Part model, mm, in its own coordinate system. Face numbers are marked on the shaded views. A direction names the side the tool comes from. Give positions to 0.01 mm unless a question says otherwise; leave off trailing zeros. Loops run counter-clockwise (first coordinate to the right, second up) from the corner with the lowest first, then second, coordinate; pieces in that order, holes last. Notation, with made-up numbers: (34.25, -8.75) -> (82.25, -8.75) arc R17 cw to (82.25, 14.25) -> close; hole circle Ø4 at (48, -8). An arc over 180 degrees is marked (long way). One line per question, with ' | ' between items.
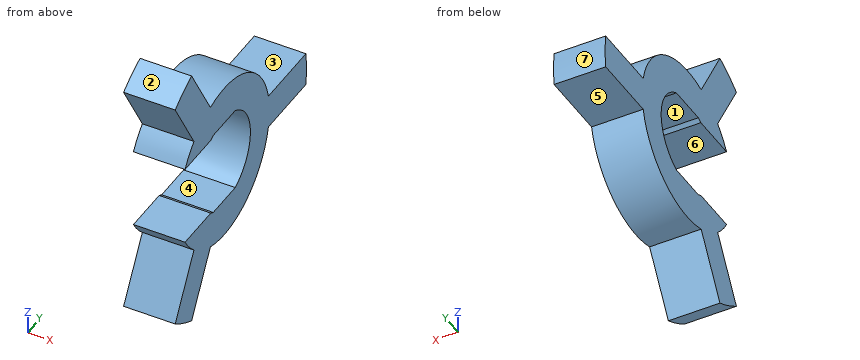
```python
from build123d import *

# Parameters (mm, degrees)
BOSS_EXTRUDE1_DEPTH = 19


with BuildPart() as part:
    # Sketch1 → Boss-Extrude1 (new body)
    with BuildSketch(Plane(origin=(0, 0, 0), x_dir=(0, 0, -1), z_dir=(1, 0, 0))):
        with BuildLine():
            Line((15.881671826, 7.35), (15.881671826, -7.35))
            ThreePointArc((15.881671826, -7.35), (15.463231756, -8.19380642), (15, -9.013878189))
            Line((15, -9.013878189), (15, -26.211447881))
            ThreePointArc((15, -26.211447881), (18.932325741, -23.528855519), (22.394280885, -20.261692516))
            Line((22.394280885, -20.261692516), (44.130028123, -32.810832035))
            ThreePointArc((44.130028123, -32.810832035), (47.62360298, -27.4955), (50.480028123, -21.812309407))
            Line((50.480028123, -21.812309407), (28.744280885, -9.263169888))
            ThreePointArc((28.744280885, -9.263169888), (26.153967194, 15.1), (6.35, 29.524862404))
            Line((6.35, 29.524862404), (6.35, 54.623141442))
            ThreePointArc((6.35, 54.623141442), (0, 54.991), (-6.35, 54.623141442))
            Line((-6.35, 54.623141442), (-6.35, 29.524862404))
            ThreePointArc((-6.35, 29.524862404), (-26.153967194, 15.1), (-28.744280885, -9.263169888))
            Line((-28.744280885, -9.263169888), (-50.480028123, -21.812309407))
            ThreePointArc((-50.480028123, -21.812309407), (-47.62360298, -27.4955), (-44.130028123, -32.810832035))
            Line((-44.130028123, -32.810832035), (-22.394280885, -20.261692516))
            ThreePointArc((-22.394280885, -20.261692516), (-18.932325741, -23.528855519), (-15, -26.211447881))
            Line((-15, -26.211447881), (-15, -9.013878189))
            ThreePointArc((-15, -9.013878189), (-15.463231756, -8.19380642), (-15.881671826, -7.35))
            Line((-15.881671826, -7.35), (-15.881671826, 7.35))
            ThreePointArc((-15.881671826, 7.35), (0, 17.5), (15.881671826, 7.35))
        make_face()
    extrude(amount=BOSS_EXTRUDE1_DEPTH)


solid = part.part
```
1) Saw through at B-B (x = 7.5). Give the cut face in (y, z), and give its area (3 significant figures).
Found:
outline: (-32.81, -44.13) arc R54.99 ccw to (-21.81, -50.48) -> (-9.26, -28.74) arc R30.2 ccw to (29.52, -6.35) -> (54.62, -6.35) arc R54.99 ccw to (54.62, 6.35) -> (29.52, 6.35) arc R30.2 ccw to (-9.26, 28.74) -> (-21.81, 50.48) arc R54.99 ccw to (-32.81, 44.13) -> (-20.26, 22.39) arc R30.2 ccw to (-26.21, 15) -> (-9.01, 15) arc R17.5 cw to (-7.35, 15.88) -> (7.35, 15.88) arc R17.5 cw to (7.35, -15.88) -> (-7.35, -15.88) arc R17.5 cw to (-9.01, -15) -> (-26.21, -15) arc R30.2 ccw to (-20.26, -22.39) -> close | area: 2,470 mm2
2) Saw through at A-A (y = -24). Give the cut face in (x, z).
Found:
outline: (0, -49.48) -> (19, -49.48) -> (19, -28.87) -> (0, -28.87) -> close; (0, -18.33) -> (19, -18.33) -> (19, -15) -> (0, -15) -> close; (0, 15) -> (19, 15) -> (19, 18.33) -> (0, 18.33) -> close; (0, 28.87) -> (19, 28.87) -> (19, 49.48) -> (0, 49.48) -> close
3) Pin check, flat tips, straight feed: P1, Ø1, axis at x = 10, z = -17.5, coming from the -Y side; P2, Ø1, axis at x = 16.5, z = 3.5, coming from the +Y side; P3, Ø3, axis at x = 14, y = 22.5, coming from the +Z side. Stop position of each tip, or through.
Found:
P1: y = -24.96 | P2: y = 54.91 | P3: z = 21.7
4) Drill centre lines: line 1 (Z direction, x = 10, y = 31); line 2 (Z direction, x = 10, y = -26.5); line 3 (Z direction, x = 3, y = -13). Where is each one in solid material? Low to high.
Found:
line 1: -6.35 to 6.35 | line 2: -48.18 to -33.2, 33.2 to 48.18 | line 3: -35.22 to -15, 15 to 35.22
5) Saw through at C-C (y = 3.5). Give the cut face in (x, z).
Found:
outline: (0, -30) -> (19, -30) -> (19, -15.88) -> (0, -15.88) -> close; (0, 15.88) -> (19, 15.88) -> (19, 30) -> (0, 30) -> close
6) Saw through at D-D (y = -11). Give the cut face in (x, z), and give its area (3 significant figures).
Found:
outline: (0, -31.75) -> (19, -31.75) -> (19, -15) -> (0, -15) -> close; (0, 15) -> (19, 15) -> (19, 31.75) -> (0, 31.75) -> close | area: 637 mm2
7) Pull direction Y, two halves, no side cores. Call the marked faces 1, 2, 3 and 4: pulls with the +Y half, pulls with the -Y half, needs draft (parallel to the pull), parting line crosses it, or undercut.
Found:
face 1: undercut | face 2: pulls with the -Y half | face 3: needs draft | face 4: undercut
8) Tool access for the marked faces 5, 6 and 7: list every direction of +Z, -Z, +X, -X, +Y, -Y with a clear straight run to the whole face (end or side of a thin tool).
Found:
face 5: -Z, +X, -X, +Y | face 6: +X, -X, -Y | face 7: +X, -X, +Y
